Source: CAD feature listing. Evaluate the final solid. Frame: model axes, mm. A direction names the side the tool comes from. Give positions to 0.01 mm unless a question says otherwise; leave off trailing zeros. Loops run counter-clockwise (first coordinate to the right, second up) from the corner with the lowest first, then second, coordinate; pieces in that order, holes last. Notation, with made-up numbers: (-6, -13.75) -> (11, -13.75) arc R22 ccw to (11, 2.25) -> close; hole circle Ø10 at (-5.75, -19). An arc over 180 degrees is marked (long way). Return JSON: item names as keys, results as strings. Group by question number.
(1) Cut plane C-C on z = 11. Return loops of the section in (x, y), then the cut area to 3 significant figures.
(2) Ray query, line 1 (X direction, y = -7, z = 16.75); line 2 (Z direction, x = 2.5, y = -1.5). Return the intervals inside material, ascending. Write a range as from..to.
(3) Cut plane D-D on y = -15.5. Return loops of the section in (x, z).
(4) Cut plane A-A on y = -6.5. Return loops of the section in (x, z).
(5) Access query for faces 1 (the face through (13, -9, 3)), 2 (the face through (0, -9, 12)). Directions: +Z, -Z, +X, -X, +Y, -Y. A direction counts if a zero-diameter tool reaches every point of the face in a straight line with its end or side. Return the directions, or none.
(6) Pin query (flat end, axial travel): pin 1 (1 mm diameter, centred on y = -5, z = 16, fed in from -X); pin 2 (3 mm diameter, centred on x = 18.5, y = -8.5, fed in from +Z); pin 3 (4 mm diameter, centred on y = -8, z = 14.5, fed in from +X). Return the tip coordinate at first contact, or that it passes through.
(7) Cut plane B-B on x = 8.25. Return loops of the section in (y, z), then the cut area to 3 significant figures.
```python
from build123d import *

# Parameters (mm, degrees)
F1_DEPTH = 18
F2_R     = 3


with BuildPart() as f1:
    # F0 (on Front) → F1 (new body)
    with BuildSketch(Plane.XZ):
        with BuildLine():
            ThreePointArc((0, 5.5), (1.610913, 1.610913), (5.5, 0))
            Line((5.5, 0), (21, 0))
            Line((21, 0), (21, 3))
            Line((21, 3), (5.5, 3))
            ThreePointArc((5.5, 3), (3.732233, 3.732233), (3, 5.5))
            Line((3, 5.5), (3, 18))
            Line((3, 18), (0, 18))
            Line((0, 18), (0, 5.5))
        make_face()
    extrude(amount=F1_DEPTH)

    # F2
    f2_edges = [f1.edges().sort_by_distance(p)[0] for p in [
        (1.5, -18, 18),
        (1.5, 0, 18),
    ]]
    fillet(f2_edges, radius=F2_R)


solid = f1.part
```
Answers:
{
 "1": {"outline": "(0, -18) -> (3, -18) -> (3, 0) -> (0, 0) -> close", "area": "54.0 mm²"},
 "2": {"line 1": "0..3", "line 2": "0.89..17.6"},
 "3": {"outline": "(0, 5.5) arc R5.5 ccw to (5.5, 0) -> (21, 0) -> (21, 3) -> (5.5, 3) arc R2.5 cw to (3, 5.5) -> (3, 17.96) -> (0, 17.96) -> close"},
 "4": {"outline": "(0, 5.5) arc R5.5 ccw to (5.5, 0) -> (21, 0) -> (21, 3) -> (5.5, 3) arc R2.5 cw to (3, 5.5) -> (3, 18) -> (0, 18) -> close"},
 "5": {"face 1": "+Z, +X, +Y, -Y", "face 2": "+Z, -Z, -X, +Y, -Y"},
 "6": {"pin 1": "x = 0", "pin 2": "z = 3", "pin 3": "x = 3"},
 "7": {"outline": "(-18, 0) -> (0, 0) -> (0, 3) -> (-18, 3) -> close", "area": "54.0 mm²"}
}
